Geometry: see drawing. Coordinates: mm, zero at the bounding-box minimum. A direction names the side the tool comes from. Round coordinates to 2 decimals unless told otherwise and drop trailing zeros. Loops run counter-clockwise (first coordinate to the right, second up) from the corner with the lowest first, then second, coordinate; pieces in that order, holes last. Notation, with made-up numbers: (61.5, 25.5) -> (81.5, 25.5) arc R13 cw to (81.5, 32.5) -> close; hole circle Ø3 at (-29, 31). An arc over 180 degrees is marked (long way). Write item = value, one per line.
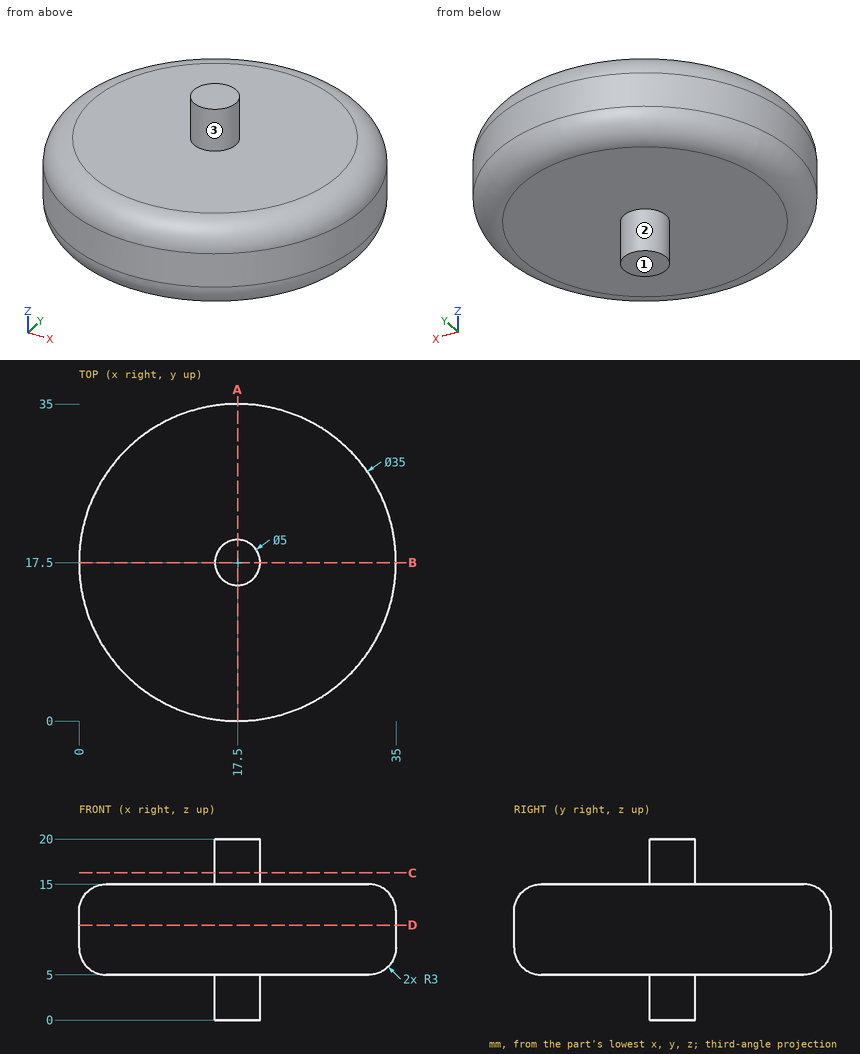
1. Line query: probe 1 along Z at (x, y) = (6, 11.5); probe 2 along Y at (x, z) = (7.5, 13.25); probe 3 along Z at (x, y) = (5, 28). Output: solid intervals per line, ascending. Write a range as from..to.
Evaluation:
probe_1 = 5..15
probe_2 = 3.47..31.53
probe_3 = 5.62..14.38
2. Section query C-C (z = 16.25). Return the cut outline in (x, y), then the cut area to 3 significant figures.
Evaluation:
outline = circle Ø5 at (17.5, 17.5)
area = 19.6 mm²
3. Set-up query: the marked faces 1, 2 and 3. Return all of +Z, -Z, +X, -X, +Y, -Y with unobstructed straight access to the full face (end or side cutting, diameter ignored); none if empty.
Evaluation:
face_1 = -Z, +X, -X, +Y, -Y
face_2 = -Z
face_3 = +Z
4. Section query D-D (z = 10.5). Return the cut outline in (x, y).
Evaluation:
outline = circle Ø35 at (17.5, 17.5)
5. Contact query for flat-ended pins moving along their axis: pin 1 Ø8 at (x, y) = (12.5, 29) entering from +Z; pin 2 Ø3 at (x, z) = (26.5, 14.5) entering from +Y; pin 3 Ø12 at (y, z) = (27.5, 8) entering from +X. Output: stop coordinate, or through.
Evaluation:
pin_1 = 15
pin_2 = 32.68
pin_3 = 34.54
6. Section query A-A (x = 17.5). Return the cut outline in (y, z).
Evaluation:
outline = (0, 8) arc R3 ccw to (3, 5) -> (15, 5) -> (15, 0) -> (20, 0) -> (20, 5) -> (32, 5) arc R3 ccw to (35, 8) -> (35, 12) arc R3 ccw to (32, 15) -> (20, 15) -> (20, 20) -> (15, 20) -> (15, 15) -> (3, 15) arc R3 ccw to (0, 12) -> close
